Job drawing, mm, ordinate dimensions from the low corner. One solid piece. Coordinates: 2 decimals unless noted, no trailing zeros. Loops run counter-clockwise (first coordinate to the right, second up) from the corner with the lowest first, then second, coordinate; pieces in that order, holes last. Notation, with made-up numbers: M -29.5,53.25 L -13.5,53.25 A27 cw -13.5,79.25 Z; hole C 13,55.25 d2. An arc over 180 degrees is marked long. Answer as a JSON object with one key per item and string values. Group by question number.
1. Saw through at D-D on z = 1. Write the cut outline in (x, y), then the cut area to 3 significant figures.
2. Drill centre lines: L1, parallel to Y at x = 12, z = 6.1; L2, parallel to Z at x = 4.25, y = 14; L3, parallel to X at y = 17.25, z = 2.25. Where is each one in solid material? Low to high.
3. Mould opens along X. For the marked faces 1, 2 and 3 say: released by +X, released by -X, zero draft, split by the parting line, or undercut.
4. Drop flat-ended pins along their axis: pin 1 Ø3 at (x, y) = (3, 10.5) entering from +Z; pin 2 Ø6.5 at (x, y) = (9, 11) entering from +Z; pin 3 Ø2 at (y, z) = (21.5, 6) entering from +X; pin 4 Ø12 at (x, y) = (20.5, 4.5) entering from +Z. Give the stop position or say it passes through.
5. Saw through at C-C on z = 4.5. Write the cut outline in (x, y).
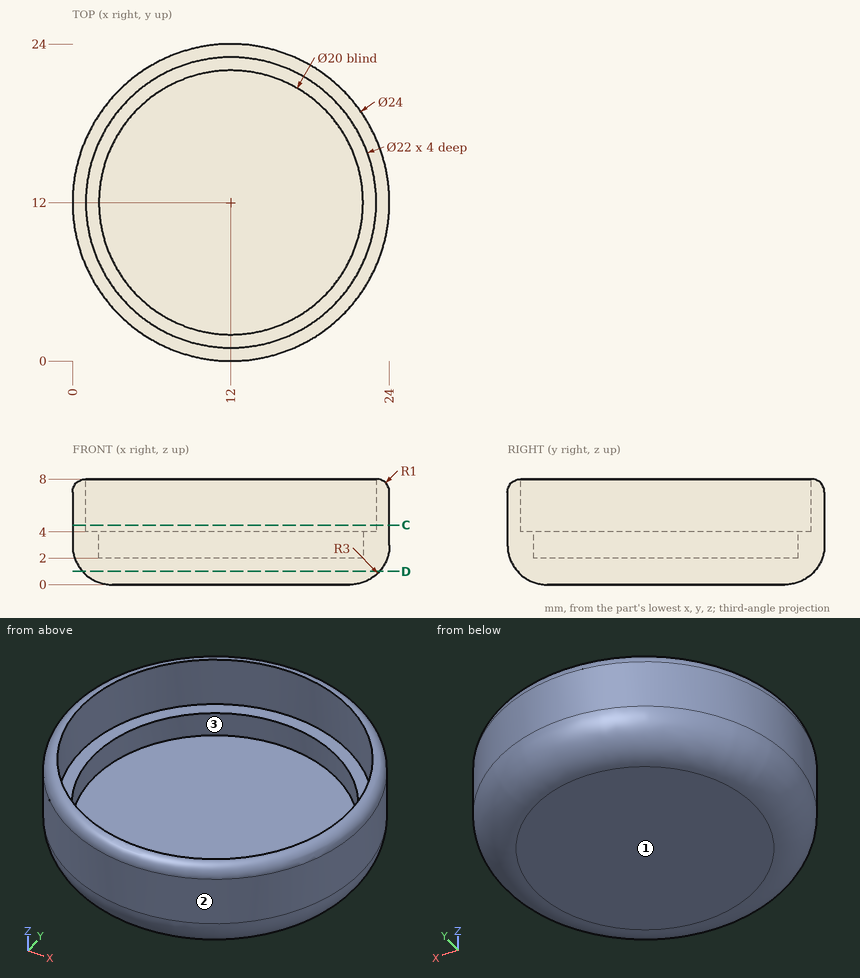
Outcome:
{
 "1": {"outline": "C 12,12 d22.47", "area": "397 mm²"},
 "2": {"L1": "y = 0 to 1, 23 to 24", "L2": "z = 0 to 2", "L3": "x = 1.32 to 3.49, 20.51 to 22.68"},
 "3": {"face 1": "zero draft", "face 2": "split by the parting line", "face 3": "undercut"},
 "4": {"pin 1": "stops at z = 4", "pin 2": "stops at z = 2", "pin 3": "stops at x = 20.47", "pin 4": "stops at z = 8"},
 "5": {"outline": "C 12,12 d24; hole C 12,12 d22"}
}
